Input: part model. Units: mm. Frame: model coordinates. Coordinates: 2 decimals unless noted, no trailing zeros. Order: outer loops, then holes, each group sorted by start corner. A loop starts at its lowest first (then second) coordinate and runs counter-clockwise, first axis right, second up.
Autodesk Inventor part; units mm, degrees
ref_plane "YZ Plane" through (0, 0, 0) normal (1, 0, 0) x (0, 1, 0)
ref_plane "XZ Plane" through (0, 0, 0) normal (0, 1, 0) x (-1, 0, 0)
ref_plane "XY Plane" through (0, 0, 0) normal (0, 0, 1) x (1, 0, 0)
sketch "Sketch2" plane through (0, 0, 0) normal (0, 1, 0) x (-1, 0, 0)
  line L0 (4, 0) -> (4, 5)
  line L1 (0, -0.9936) -> (0, 4.4305)
  line L2 (4, 5) -> (4, 0)
  line L3 (1, 1.2185) -> (1, 1.7185)
  line L4 (1, 1.2185) -> (2, 0)
  line L5 (2, 0) -> (4, 0)
  line L6 (4, 5) -> (3, 5)
  line L7 (3, 5) -> (1, 1.7185)
  point P0 (0, 0)
  dimension "d4" = 5
  dimension "d16" = 1
  dimension "d18" = 2
  dimension "d24" = 1
  dimension "d25" = 4
revolve "Revolution2" add sketch "Sketch2" angle 360 about axis through (0, 0, -0.9936) along (0, 0, 1)
fillet "Fillet3" radius 0.2 2 edges at (1, 0, 1.7185) (1, 0, 1.2185)
properties part number "nozzle_small" material "Glass"
Item 1: Pin query (flat end, axial travel): pin 1 Ø2.5 at (x, y) = (0, 0) entering from +Z; pin 2 Ø3 at (x, z) = (-3, 3) entering from -Y; pin 3 Ø1.5 at (x, z) = (-3, 3) entering from +Y. Return the tip coordinate at first contact, or that it passes through.
Response values:
pin 1: stops at z = 2.13
pin 2: stops at y = -3.71
pin 3: stops at y = 3.31
Item 2: Cut plane C-C on z = 4.1. Return loops of the section in (x, y), then the cut area to 3 significant figures.
Response values:
outline: circle Ø8 at (0, 0); hole circle Ø4.9 at (0, 0)
area: 31.4 mm2
Item 3: Cut plane B-B on y = 3.75. Return loops of the section in (x, z), then the cut area to 3 significant figures.
Response values:
outline: (-1.39, 0) - (1.39, 0) - (1.39, 5) - (-1.39, 5) - close
area: 13.9 mm2
Item 4: Cut plane A-A on z = 1.5. Return loops of the section in (x, y).
Response values:
outline: circle Ø8 at (0, 0); hole circle Ø2 at (0, 0)
Item 5: Ray query, probe 1 along Y at (x, z) = (0, 1.5); probe 2 along Y at (x, z) = (-0.5, 2.05). Return the intervals inside material, ascending.
Response values:
probe 1: y = -4 to -1, 1 to 4
probe 2: y = -3.97 to -1.09, 1.09 to 3.97
Item 6: Draft query along X for faces 1 (the face through (2, 1, 0)), 2 (the face through (0.867, 3.905, 2.535)), 3 (the face through (0.3, 1.34, 2.33)). Return one class per face: pulls with the +X half, pulls with the -X half, needs draft (parallel to the pull), parting line crosses it, or undercut.
Response values:
face 1: needs draft
face 2: parting line crosses it
face 3: undercut
